The figure shows three views and two pictorial views of one solid part (mm, origin at its lowest corner). Answer the questions. Round coordinates to 2 decimals unless told otherwise and drop trailing zeros. Order: outer loops, then holes, each group sorted by start corner. A loop starts at its lowest first (then second) coordinate and runs counter-clockwise, first axis right, second up. Notation, with made-up numbers: M -20,53.25 L 34,53.25 A25 ccw 34,91.25 Z; hole C 7.25,31 d7. An arc over 180 degrees is marked long. Answer as CSV lines item,"result".
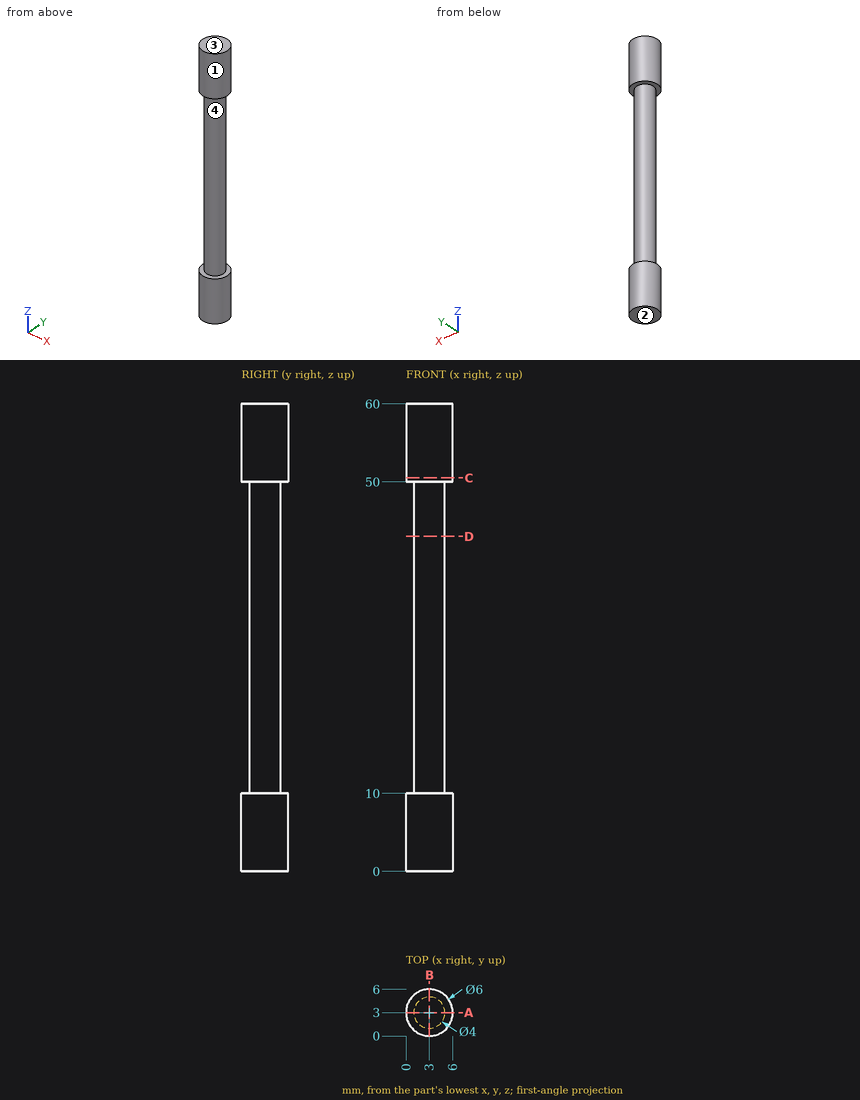
Item 1: Determine the mould class of the marked faces 1, 2, 3 and 4 for opening direction Z: +Z half, -Z half, draft (parallel to the pull), parting line (faces both ways), or undercut.
Ans:
face 1,"draft"
face 2,"-Z half"
face 3,"+Z half"
face 4,"undercut"
Item 2: Find the intervals of material crossed by probe 1 along Z at (x, y) = (1.5, 4.45); probe 2 along X at (y, z) = (2.7, 3); probe 3 along Y at (x, z) = (4.55, 38), in increasing order. Write a range as [from, to].
Ans:
probe 1,"[0, 10], [50, 60]"
probe 2,"[0.02, 5.98]"
probe 3,"[1.74, 4.26]"
Item 3: A cutting plane is placed at A-A, the plane y = 3. Determine the outline of the cut face in (x, z), and give its area (3 significant figures).
Ans:
outline,"M 0,0 L 6,0 L 6,10 L 5,10 L 5,50 L 6,50 L 6,60 L 0,60 L 0,50 L 1,50 L 1,10 L 0,10 Z"
area,"280 mm2"
Item 4: A cutting plane is placed at C-C, the plane z = 50.5. Determine the outline of the cut face in (x, y).
Ans:
outline,"C 3,3 d6"
Item 5: A cutting plane is placed at D-D, the plane z = 43. Determine the outline of the cut face in (x, y).
Ans:
outline,"C 3,3 d4"
Item 6: Flat-ended cylindrical pins translate along their axes: pin 1 (1 mm diameter, centred on y = 3.5, z = 19.5, fed in from -X); pin 2 (3 mm diameter, centred on x = 4, z = 20.5, fed in from -Y). Find the tip coordinate at first contact, or state that the pin passes through.
Ans:
pin 1,"x = 1"
pin 2,"y = 1"
